CAD build for the part. Positions are in the model's coordinates, mm. A direction names the side the tool comes from. Coordinates: 2 decimals unless noted, no trailing zeros. Loops run counter-clockwise (first coordinate to the right, second up) from the corner with the lowest first, then second, coordinate; pieces in that order, holes last. Notation, with made-up numbers: (88, -26) -> (136, -26) arc R13 ccw to (136, -6) -> close; hole circle Ø9 at (69.5, 49). An arc over 180 degrees is marked (long way). Answer as CSV lines item,"result". Start each with the question number.
```python
from build123d import *

# Parameters (mm, degrees)
ESQUISSE1_W        = 125
ESQUISSE1_H        = 30.99
BOSS_EXTRU_1_DEPTH = 2
CONG_1_R           = 15
ESQUISSE2_R        = 4.25
ESQUISSE2_R_2      = 1.75
BOSS_EXTRU_2_DEPTH = 9


with BuildPart() as part:
    # Esquisse1 → Boss.-Extru.1 (new body)
    with BuildSketch(Plane.XY):
        with Locations((-62.5, 15.495)):
            Rectangle(ESQUISSE1_W, ESQUISSE1_H)
    extrude(amount=BOSS_EXTRU_1_DEPTH)

    # Congé1
    cong_1_edges = [part.edges().sort_by_distance(p)[0] for p in [
        (0, 0, 1),
        (-125, 0, 1),
        (-125, 30.99, 1),
        (0, 30.99, 1),
    ]]
    fillet(cong_1_edges, radius=CONG_1_R)

    # Esquisse2 → Boss.-Extru.2 (add)
    # profile 1 of 2: a face of its own
    with BuildSketch(Plane.XY.offset(2)):
        with Locations((-95, 16.75)):
            Circle(ESQUISSE2_R)
        with Locations((-95, 16.75)):
            Circle(ESQUISSE2_R_2, mode=Mode.SUBTRACT)
    # profile 2 of 2: a face of its own
    with BuildSketch(Plane.XY.offset(2)):
        with Locations((-30, 16.75)):
            Circle(ESQUISSE2_R)
        with Locations((-30, 16.75)):
            Circle(ESQUISSE2_R_2, mode=Mode.SUBTRACT)
    extrude(amount=BOSS_EXTRU_2_DEPTH)


solid = part.part
```
Q1. Saw through at B-B (x = -30). List the corners of the cut face in (y, z).
Q2. Probe probe 1 along X at (y, z) = (16, 10.25); probe 2 along Y at (x, z) = (-30, 6.25); probe 3 along Z at (x, y) = (-21, 24). List the from-to ranges inside material, lowest first. Write a range as from..to.
Q3. Which spindle directions (+Z, -Z, +X, -X, +Y, -Y) get a long thin tool onto all of the face, cutting with end or side? Do faces 1 (the flat face through (-63, 0, 1)), 2 (the flat face through (-30, 17, 2)). Say none if no direction does.
Q4. Saw through at A-A (z = 4.75). List the corners of the cut face in (x, y), and give its area (3 significant figures).
Q5. Pin check, flat tips, straight feed: pin 1 Ø4 at (y, z) = (13, 8) entering from +X; pin 2 Ø4 at (y, z) = (17.5, 9) entering from +X; pin 3 Ø4 at (x, y) = (-67, 19) entering from +Z. Stop position of each tip, or through.
Q6. Two-plate mould, pull along Y, no slides. Class faces 3 (the cylindrical face through (-120.72, 4.51, 1.01)), 4 (the flat face through (-63, 16, 0)), 5 (the cylindrical face through (-31.29, 17.93, 6.44)): pulls with the +Y half, pulls with the -Y half, needs draft (parallel to the pull), parting line crosses it, or undercut.
Q7. Saw through at D-D (x = -84.5). List the corners of the cut face in (y, z).
Q8. Saw through at C-C (y = 6.5). List the corners of the cut face in (x, z), and give its area (3 significant figures).
Ans:
1,outline,"(0, 0) -> (30.99, 0) -> (30.99, 2) -> (21, 2) -> (21, 11) -> (18.5, 11) -> (18.5, 2) -> (15, 2) -> (15, 11) -> (12.5, 11) -> (12.5, 2) -> (0, 2) -> close"
2,probe 1,"x = -99.18..-96.58, -93.42..-90.82, -34.18..-31.58, -28.42..-25.82"
2,probe 2,"y = 12.5..15, 18.5..21"
2,probe 3,"z = 0..2"
3,face 1,"+Z, -Z, +X, -X, -Y"
3,face 2,"+Z"
4,outline,"circle Ø8.5 at (-95, 16.75); circle Ø8.5 at (-30, 16.75); hole circle Ø3.5 at (-95, 16.75); hole circle Ø3.5 at (-30, 16.75)"
4,area,"94.2 mm²"
5,pin 1,"stops at x = -26.13"
5,pin 2,"stops at x = -25.75"
5,pin 3,"stops at z = 2"
6,face 3,"pulls with the -Y half"
6,face 4,"needs draft"
6,face 5,"undercut"
7,outline,"(0, 0) -> (30.99, 0) -> (30.99, 2) -> (0, 2) -> close"
8,outline,"(-122.36, 0) -> (-2.64, 0) -> (-2.64, 2) -> (-122.36, 2) -> close"
8,area,"239 mm²"
